Input: part model. Units: mm. Frame: model coordinates. A direction names the side the tool comes from. Give positions to 0.01 mm unless a question says otherwise; leave off trailing zeros. Loops run counter-clockwise (first coordinate to the right, second up) from the corner with the lowest first, then second, coordinate; pieces in that order, holes last. Notation, with made-up numbers: (-40, -37.75) - (9, -37.75) arc R22 ccw to (9, -4.75) - close; hole circle Ø8 at (-7.75, -20). An arc over 180 degrees is marked (long way). One line per item, written item: value.
from build123d import *

# Parameters (mm, degrees)
EXTRUDE002_DEPTH = 2
EXTRUDE_DEPTH    = 3
CHAMFER_SIZE     = 2
CHAMFER001_SIZE  = 0.5
EXTRUDE001_DEPTH = 3


with BuildPart() as extrude002:
    # Sketch002 (on Face10 of Extrude001) → Extrude002 (new body)
    with BuildSketch(Plane.XY.offset(6)):
        with BuildLine():
            ThreePointArc((-4.5, -10), (0, -10.965856), (4.5, -10))
            Line((4.5, -7), (4.5, -10))
            ThreePointArc((-4.5, -7), (0, -8.321658), (4.5, -7))
            Line((-4.5, -7), (-4.5, -10))
        make_face()
    extrude(amount=EXTRUDE002_DEPTH)


with BuildPart() as chamfer001:
    # Sketch → Extrude (new body)
    with BuildSketch(Plane.XY):
        with BuildLine():
            Line((9.75, 28), (9.75, 0))
            Line((9.75, -3), (9.75, 0))
            Line((7.5, -3), (9.75, -3))
            Line((7.5, -8), (7.5, -3))
            ThreePointArc((-7.5, -8), (0, -10.965856), (7.5, -8))
            Line((-7.5, -3), (-7.5, -8))
            Line((-9.75, -3), (-7.5, -3))
            Line((-9.75, 0), (-9.75, -3))
            Line((-9.75, 0), (-9.75, 28))
            ThreePointArc((9.75, 28), (0, 31.576886), (-9.75, 28))
        make_face()
        with BuildLine():
            ThreePointArc((7.25, 20.93706), (0, 25), (-7.25, 20.93706))
            Line((-7.25, 20.93706), (-7.25, 12.06294))
            ThreePointArc((-7.25, 12.06294), (-6.772193, 11.363133), (-6.227082, 10.714376))
            Line((-3.415063, 15.584937), (-6.227082, 10.714376))
            ThreePointArc((0.915063, 13.084936), (0, 16.5), (-3.415063, 15.584937))
            Line((0.915063, 13.084936), (-1.896956, 8.214376))
            ThreePointArc((-1.896956, 8.214376), (3.296457, 8.665246), (7.25, 12.06294))
            Line((7.25, 20.93706), (7.25, 12.06294))
        make_face(mode=Mode.SUBTRACT)
    extrude(amount=EXTRUDE_DEPTH)

    # Chamfer
    chamfer_edges = [chamfer001.edges().sort_by_distance(p)[0] for p in [
        (-9.75, 14, 0),
        (9.75, 14, 0),
        (9.75, -1.5, 0),
        (-9.75, -1.5, 0),
    ]]
    chamfer(chamfer_edges, length=CHAMFER_SIZE)

    # Chamfer001
    chamfer001_edges = [chamfer001.edges().sort_by_distance(p)[0] for p in [
        (0, 31.576886, 3),
        (-4.821073, 13.149656, 3),
    ]]
    chamfer(chamfer001_edges, length=CHAMFER001_SIZE)


with BuildPart() as fusion:
    # Sketch001 (on Face4 of Chamfer) → Extrude001 (new body)
    with BuildSketch(Plane.XY.offset(3)):
        with BuildLine():
            Line((9.75, 0), (-9.75, 0))
            Line((-9.75, 0), (-9.75, -3))
            Line((-9.75, -3), (-7.5, -3))
            Line((-7.5, -3), (-7.5, -8))
            ThreePointArc((-7.5, -8), (0, -10.965856), (7.5, -8))
            Line((7.5, -3), (7.5, -8))
            Line((9.75, -3), (7.5, -3))
            Line((9.75, 0), (9.75, -3))
        make_face()
    extrude(amount=EXTRUDE001_DEPTH)

    # Fusion: union Extrude002, Chamfer001
    add(extrude002.part)
    add(chamfer001.part)


solid = fusion.part
Item 1: Draft query along Y for faces 4 (the face through (-0.471, 10.684, 1.232)), 5 (the face through (-8.74, 13.44, 0.99)), 6 (the face through (0, 0, 4)). Return one class per face: pulls with the +Y half, pulls with the -Y half, needs draft (parallel to the pull), parting line crosses it, or undercut.
Verdict:
face 4: undercut
face 5: needs draft
face 6: pulls with the +Y half
Item 2: Section D-D, the plane z = 1. Output: boundary loops of the cut face in (x, y).
Verdict:
outline: (-8.75, -3) - (-7.5, -3) - (-7.5, -8) arc R10.97 ccw to (7.5, -8) - (7.5, -3) - (8.75, -3) - (8.75, 28.78) arc R15.08 ccw to (-8.75, 28.78) - close; hole (-7.25, 12.06) arc R8.5 ccw to (-6.23, 10.71) - (-3.42, 15.58) arc R2.5 cw to (0.92, 13.08) - (-1.9, 8.21) arc R8.5 ccw to (7.25, 12.06) - (7.25, 20.94) arc R8.5 ccw to (-7.25, 20.94) - close
Item 3: Section B-B, the plane z = 4.25. Output: boundary loops of the cut face in (x, y).
Verdict:
outline: (-9.75, -3) - (-7.5, -3) - (-7.5, -8) arc R10.97 ccw to (7.5, -8) - (7.5, -3) - (9.75, -3) - (9.75, 0) - (-9.75, 0) - close
Item 4: Material intervals for L1, parallel to Y at x = 0, z = 1.75; L2, parallel to X at y = 18.5, z = 2.5; L3, parallel to Y at x = 1, z = 0.5, sorted ascending.
Verdict:
L1: y = -10.97 to 8, 11.5 to 16.5, 25 to 31.58
L2: x = -9.75 to -7.25, 7.25 to 9.75
L3: y = -10.92 to 8.06, 13.25 to 15.42, 24.94 to 31.54
Item 5: Access query for faces 1 (the face through (-4.5, -8, 7)), 2 (the face through (7.25, 17, 1)), 3 (the face through (-7.5, -5, 3)). Directions: +Z, -Z, +X, -X, +Y, -Y. A direction counts if a zero-diameter tool reaches every point of the face in a straight line with its end or side. Return the directions, or none.
Verdict:
face 1: +Z, -X, +Y, -Y
face 2: +Z, -Z
face 3: +Z, -Z, -X, -Y
Item 6: Section A-A, the plane y = 24. Output: boundary loops of the cut face in (x, z).
Verdict:
outline: (-9.75, 2) - (-7.75, 0) - (-4, 0) - (-4, 3) - (-9.75, 3) - close; (4, 0) - (7.75, 0) - (9.75, 2) - (9.75, 3) - (4, 3) - close
Item 7: Section C-C, the plane y = -0.5. Output: boundary loops of the cut face in (x, z), and give its area (3 significant figures).
Verdict:
outline: (-9.75, 2) - (-7.75, 0) - (7.75, 0) - (9.75, 2) - (9.75, 6) - (-9.75, 6) - close
area: 113 mm^2
Item 8: Pin query (flat end, axial travel): P1, Ø2.5, axis at y = 17.5, z = 1, coming from the +X side; P2, Ø2.5, axis at x = 8, z = 2.5, coming from the -Y side; P3, Ø1.5, axis at y = -5, z = 1.5, coming from the -X side; P4, Ø1.5, axis at y = -6, z = 4, coming from the +X side. Return the tip coordinate at first contact, or that it passes through.
Verdict:
P1: stops at x = 9.75
P2: stops at y = -8.64
P3: stops at x = -7.5
P4: stops at x = 7.5
